For this review, take the finished solid that the model builds, in its own axes (mm). Round coordinates to 2 decimals unless told otherwise and drop trailing zeros. Write each loop counter-clockwise with the first axis right and the second up, starting at its lowest first coordinate (ties: lowest second). Pieces come first, ordered by that corner, then holes. Notation, with made-up numbers: M 75.25,76 L 133.25,76 A14 ccw 133.25,91 Z; hole C 21,63.5 d1. An arc over 180 degrees is marked long. One line per question, with ' | ' between items.
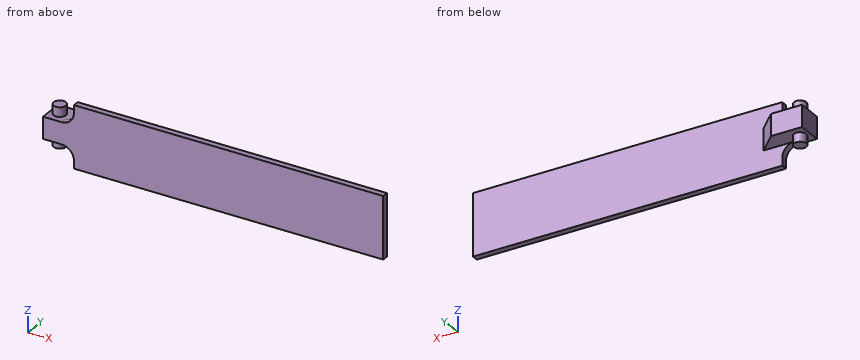
```python
from build123d import *

# Parameters (mm, degrees)
SKETCH2_W           = 10
SKETCH2_H           = 7
BOSS_EXTRUDE1_DEPTH = 8
SKETCH3_R           = 2
BOSS_EXTRUDE2_DEPTH = 3
SKETCH4_W           = 20
SKETCH4_H           = 2
BOSS_EXTRUDE3_DEPTH = 100
CHAMFER1_SIZE       = 6
FILLET1_R           = 4


with BuildPart() as part:
    # Sketch2 → Boss-Extrude1 (new body)
    with BuildSketch(Plane(origin=(0, 0, 0), x_dir=(1, 0, 0), z_dir=(0, 1, 0))):
        with Locations((5, 0)):
            Rectangle(SKETCH2_W, SKETCH2_H)
    extrude(amount=BOSS_EXTRUDE1_DEPTH)

    # Sketch3 → Boss-Extrude2 (add)
    with BuildSketch(Plane.XY.offset(3.5)):
        with Locations((3.01, 4)):
            Circle(SKETCH3_R)
    boss_extrude2 = extrude(amount=BOSS_EXTRUDE2_DEPTH)

    # Mirror1: Boss-Extrude2 across plane
    add(boss_extrude2.mirror(Plane.XY))

    # Sketch4 → Boss-Extrude3 (add)
    with BuildSketch(Plane(origin=(10, 0, 0), x_dir=(0, 0, -1), z_dir=(1, 0, 0))):
        with Locations((0, 1)):
            Rectangle(SKETCH4_W, SKETCH4_H)
    extrude(amount=BOSS_EXTRUDE3_DEPTH)

    # Chamfer1
    chamfer1_edges = [part.edges().sort_by_distance(p)[0] for p in [
        (10, 2, 0),
    ]]
    chamfer(chamfer1_edges, length=CHAMFER1_SIZE - 0.0001)  # a hair under: the kernel refuses the full size

    # Fillet1
    fillet1_edges = [part.edges().sort_by_distance(p)[0] for p in [
        (10, 1, -3.5),
        (10, 1, 3.5),
    ]]
    fillet(fillet1_edges, radius=FILLET1_R)


solid = part.part
```
Item 1: Insertion check: pin 1 Ø4 at (x, y) = (11.5, 5) entering from +Z; pin 2 Ø1.2 at (x, y) = (2, 4.5) entering from -Z; pin 3 Ø5 at (x, z) = (49, 2) entering from +Y. Each pin has a flat end and moves straight along its axis. Give the tip position at first contact, or say it passes through.
Results:
pin 1: z = 3.5 | pin 2: z = -6.5 | pin 3: y = 2
Item 2: Take a section at D-D (z = 4.5). Write out the cut boundary in (x, y), then the cut area to 3 significant figures.
Results:
outline: C 3.01,4 d4; M 8.65,0 L 110,0 L 110,2 L 8.65,2 Z | area: 215 mm2
Item 3: To check wall thickness, follow line 1 along Z through (x, y) = (10, 4.5); line 2 along Y through (x, z) = (98, 0.75); line 3 along X through (y, z) = (2.5, -2.75). State the ranges of each line that lie inside material, in increasing order. Write a range as from..to.
Results:
line 1: -3.5..3.5 | line 2: 0..2 | line 3: 0..15.5
Item 4: Take a section at C-C (y = 4). Write out the cut boundary in (x, z), then the cut area to 3 significant figures.
Results:
outline: M 0,-3.5 L 1.01,-3.5 L 1.01,-6.5 L 5.01,-6.5 L 5.01,-3.5 L 14,-3.5 L 14,3.5 L 5.01,3.5 L 5.01,6.5 L 1.01,6.5 L 1.01,3.5 L 0,3.5 Z | area: 122 mm2
Item 5: Take a section at A-A (x = 3.01). Write out the cut boundary in (y, z), then the cut area to 3 significant figures.
Results:
outline: M 0,-3.5 L 2,-3.5 L 2,-6.5 L 6,-6.5 L 6,-3.5 L 8,-3.5 L 8,3.5 L 6,3.5 L 6,6.5 L 2,6.5 L 2,3.5 L 0,3.5 Z | area: 80.0 mm2
